Source: CAD feature listing. Evaluate the final solid. Frame: model axes, mm. A direction names the side the tool comes from. Give positions to 0.01 mm unless a question says otherwise; leave off trailing zeros. Write each loop counter-clockwise with the first axis right and the second up, starting at its lowest first coordinate (ties: lowest second). Pieces come first, ordered by that corner, then holes. Notation, with made-up numbers: (1, 69) - (8, 69) arc R9 ccw to (8, 73) - close; hole circle Ø2 at (82.5, 83). An arc over 180 degrees is marked (long way). One line per question, with ' | ' between items. Start each with the question number.
(1) Draft query along X for faces 4 (the flat face through (60, 0, 42.875)), 5 (the flat face through (41.275, -1, 5)), 6 (the flat face through (1, -36, 9.525)), 7 (the flat face through (22.225, -17, 18)). Return one class per face: +X half, -X half, draft (parallel to the pull), parting line (faces both ways), or undercut.
(2) Section B-B, the plane x = 77. Return loops of the section in (y, z) (3 decimals).
(3) Ray query, line 1 (Y direction, x = 54, z = 54); line 2 (Y direction, x = -14.5, z = 39); line 3 (Z direction, x = 92, y = 22.5) (3 decimals). Return the intervals inside material, ascending. Write a range as [from, to].
(4) Access query for faces 1 (the flat face through (89, 0, 38.1)), 2 (the cylindrical face through (31.361, -16.791, 50.767)), 3 (the flat face through (-4, 7.938, 36)). Directions: +Z, -Z, +X, -X, +Y, -Y. A direction counts if a zero-diameter tool reaches every point of the face in a straight line with its end or side. Return the directions, or none.
(5) Pin query (flat end, axial travel): pin 1 (1 mm diameter, centred on y = 12, z = 54.5, fed in from -X); pin 2 (8.5 mm diameter, centred on y = 17.5, z = 18, fed in from -X) (3 decimals); pin 3 (1.5 mm diameter, centred on y = -21.5, z = 50.5, fed in from +X); pin 4 (19 mm diameter, centred on y = -17, z = 15.5, fed in from -X) (3 decimals). Return the tip coordinate at first contact, or that it passes through.
(6) Section C-C, the plane z = 0. Return loops of the section in (x, y) (3 decimals).
(7) Section A-A, the plane y = -32. Return loops of the section in (x, z) (3 decimals), plus the area to 3 significant figures.
```python
from build123d import *

# Parameters (mm, degrees)
F1_DEPTH = 63.5
F0_W     = 25.4
F0_H     = 19.05
F2_DEPTH = 25.4
F3_DEPTH = 7.9375


with BuildPart() as f1:
    # F0 (on Front) → F1 (new body, symmetric)
    with BuildSketch(Plane.XZ):
        Polygon((-41.275, 9.525), (-41.275, -9.525), (41.275, -9.525), (41.275, 9.525), (22.225, 9.525), align=None)
    extrude(amount=F1_DEPTH, both=True)

    # F0 (on Front) → F2 (join, symmetric)
    with BuildSketch(Plane.XZ):
        with Locations((75.5235318422, 52.4002)):
            Rectangle(F0_W, F0_H)
        with BuildLine():
            Line((22.225, 9.525), (41.275, 9.525))
            Line((41.275, 9.525), (41.275, 27.2153939429))
            ThreePointArc((41.275, 27.2153939429), (45.0386370244, 37.4784593657), (54.5449857479, 42.8752))
            Line((54.5449857479, 42.8752), (62.8235318422, 42.8752))
            Line((62.8235318422, 42.8752), (62.8235318422, 61.9252))
            Line((62.8235318422, 61.9252), (53.2789551181, 61.9252))
            ThreePointArc((53.2789551181, 61.9252), (31.1216321343, 50.5022935057), (22.225, 27.2153939429))
            Line((22.225, 27.2153939429), (22.225, 9.525))
        make_face()
    extrude(amount=F2_DEPTH, both=True)

    # F0 (on Front) → F3 (join, symmetric)
    with BuildSketch(Plane.XZ):
        with BuildLine():
            add(Edge.make_bspline(
                [(-41.275, 9.525), (-40.8366508782, 51.8352910876), (-5.1678125747, 62.6129284501), (53.2789551181, 61.9252)],
                knots=[0, 0, 0, 0, 108.1028740992, 108.1028740992, 108.1028740992, 108.1028740992], degree=3))
            Line((-41.275, 9.525), (22.225, 9.525))
            Line((22.225, 9.525), (22.225, 27.2153939429))
            ThreePointArc((22.225, 27.2153939429), (31.1216321343, 50.5022935057), (53.2789551181, 61.9252))
        make_face()
    extrude(amount=F3_DEPTH, both=True)

    # F0 (on Front) → F4 (revolve)
    with BuildSketch(Plane.XZ):
        Polygon((88.2235318422, 66.675), (88.2235318422, 61.9252), (88.2235318422, 42.8752), (88.2235318422, 38.1), (113.6235318422, 38.1), (113.6235318422, 66.675), align=None)
    revolve(axis=Axis((88.2235318422, 0, 52.3875), (0, 0, 1)))


solid = f1.part
```
Check sheet entries:
1) face 4: undercut | face 5: +X half | face 6: draft | face 7: -X half
2) outline: (-25.4, 42.875) - (-22.786, 42.875) - (-22.786, 38.1) - (22.786, 38.1) - (22.786, 42.875) - (25.4, 42.875) - (25.4, 61.925) - (22.786, 61.925) - (22.786, 66.675) - (-22.786, 66.675) - (-22.786, 61.925) - (-25.4, 61.925) - close
3) line 1: [-25.4, 25.4] | line 2: [-7.94, 7.94] | line 3: [38.1, 66.675]
4) face 1: -Z, +X, +Y, -Y | face 2: +Z, -X, -Y | face 3: +Z, -X, +Y
5) pin 1: x = 34.74 | pin 2: x = 22.225 | pin 3: x = 102.87 | pin 4: x = -41.275
6) outline: (-41.275, -63.5) - (41.275, -63.5) - (41.275, 63.5) - (-41.275, 63.5) - close
7) outline: (-41.275, -9.525) - (41.275, -9.525) - (41.275, 9.525) - (-41.275, 9.525) - close | area: 1,570 mm²
